Input: part model. Units: mm. Frame: model coordinates. A direction names the side the tool comes from. Coordinates: 2 decimals unless noted, no trailing zeros. Order: outer loops, then holes, each group sorted by start corner. A loop starts at its lowest first (then second) coordinate and runs counter-clockwise, first axis right, second up. Notation, with made-up numbers: (75, 37.25) -> (127, 37.25) arc R22 cw to (127, 67.25) -> close; hole circle Ø3 at (-18, 11.25). An arc over 180 degrees is marked (long way). One line per question, with ' | ' between items.
```python
from build123d import *

# Parameters (mm, degrees)
F0_R      = 25
F1_DEPTH  = 47
F2_R      = 32.5
F3_DEPTH  = 160
F4_R      = 25
F5_DEPTH  = 47
F7_W      = 60.588232
F7_H      = 10
F8_DEPTH  = 25
F9_W      = 55.500018
F9_H      = 10
F10_DEPTH = 25
F11_R     = 4
F12_DEPTH = 25
F13_R     = 4
F14_DEPTH = 92
F15_R     = 5
F16_DEPTH = 18.5
F17_SIZE  = 1.5


with BuildPart() as f1:
    # F0 (on Front) → F1 (new body)
    with BuildSketch(Plane.XZ):
        Circle(F0_R)
    extrude(amount=-F1_DEPTH)

    # F2 (on face) → F3 (join)
    with BuildSketch(Plane(origin=(0, 47, 0), x_dir=(-1, 0, 0), z_dir=(0, 1, 0))):
        Circle(F2_R)
    extrude(amount=F3_DEPTH)

    # F4 (on face) → F5 (join)
    with BuildSketch(Plane(origin=(0, 207, 0), x_dir=(-1, 0, 0), z_dir=(0, 1, 0))):
        Circle(F4_R)
    extrude(amount=F5_DEPTH)

    # F7 (on offset) → F8 (cut)
    with BuildSketch(Plane.XY.offset(17)):
        with Locations((8.858869, 15)):
            Rectangle(F7_W, F7_H)
    extrude(amount=F8_DEPTH, mode=Mode.SUBTRACT)

    # F9 (on offset) → F10 (cut)
    with BuildSketch(Plane.XY.offset(17)):
        with Locations((1.929622, 239)):
            Rectangle(F9_W, F9_H)
    extrude(amount=F10_DEPTH, mode=Mode.SUBTRACT)

    # F11 (on Front) → F12 (cut)
    with BuildSketch(Plane.XZ):
        Circle(F11_R)
    extrude(amount=-F12_DEPTH, mode=Mode.SUBTRACT)

    # F13 (on Top) → F14 (cut)
    with BuildSketch(Plane.XY):
        with Locations((0, 74.5)):
            Circle(F13_R)
        with Locations((0, 179.5)):
            Circle(F13_R)
    extrude(amount=F14_DEPTH, mode=Mode.SUBTRACT)

    # F15 (on Front) → F16 (cut)
    with BuildSketch(Plane.XZ):
        Circle(F15_R)
    extrude(amount=-F16_DEPTH, mode=Mode.SUBTRACT)

    # F17
    f17_edges = [f1.edges().sort_by_distance(p)[0] for p in [
        (-25, 0, 0),
        (25, 254, 0),
    ]]
    chamfer(f17_edges, length=F17_SIZE)


solid = f1.part
```
1. Cut plane B-B, the plane y = 133. Return loops of the section in (x, z), and give its area (3 significant figures).
Recorded:
outline: circle Ø65 at (0, 0) | area: 3,320 mm^2
2. Mould query, pull axis Z, two halves, no side actions, for faces 1 (the face through (-0.521, 183.466, 16.027)), 2 (the face through (0, 25, 0)), 3 (the face through (-5.42, 23.932, -24.406)). Classes: released by +Z, released by -Z, zero draft, split by the parting line, or undercut.
Recorded:
face 1: zero draft | face 2: undercut | face 3: split by the parting line
3. Cut plane C-C, the plane y = 179.5. Return loops of the section in (x, z).
Recorded:
outline: (-4, 0) -> (-4, 32.25) arc R32.5 ccw (long way) to (4, 32.25) -> (4, 0) -> close
4. Cut plane A-A, the plane y = 33. Return loops of the section in (x, z), and give its area (3 significant figures).
Recorded:
outline: circle Ø50 at (0, 0) | area: 1,960 mm^2
5. Access query for faces 4 (the face through (0, 75, 0)), 5 (the face through (-1.08, 9.12, -4.88)), 6 (the face through (0, 234, 20)). Directions: +Z, -Z, +X, -X, +Y, -Y. A direction counts if a zero-diameter tool reaches every point of the face in a straight line with its end or side. Return the directions, or none.
Recorded:
face 4: +Z | face 5: -Y | face 6: +Z, +X, -X
6. Pin query (flat end, axial travel): pin 1 Ø2 at (x, z) = (24.5, -14.5) entering from -Y; pin 2 Ø6.5 at (x, y) = (0, 179.5) entering from +Z; pin 3 Ø1 at (y, z) = (94.5, 17.5) entering from +X. Return the tip coordinate at first contact, or that it passes through.
Recorded:
pin 1: stops at y = 47 | pin 2: stops at z = 0 | pin 3: stops at x = 27.7
7. Ray query, line 1 (Y direction, x = 0, z = 11); line 2 (Z direction, x = 0, y = 13); line 3 (Z direction, x = 0, y = 5). Return the intervals inside material, ascending. Write a range as [from, to].
Recorded:
line 1: y = [0, 70.5], [78.5, 175.5], [183.5, 254] | line 2: z = [-25, -5], [5, 17] | line 3: z = [-25, -5], [5, 25]
